from build123d import *

# Parameters (mm, degrees)
SKETCH1_R           = 3.5687
SKETCH1_R_2         = 2
BOSS_EXTRUDE1_DEPTH = 4.191
SKETCH5_R           = 2
SKETCH5_R_2         = 1.143
BOSS_EXTRUDE2_DEPTH = 0.2226
SKETCH6_R           = 0.5334
BOSS_EXTRUDE3_DEPTH = 1.524


with BuildPart() as part:
    # Sketch1 → Boss-Extrude1 (new body)
    with BuildSketch(Plane.XY.offset(-7.032965862)):
        with Locations((-5.5, 0)):
            Circle(SKETCH1_R)
        with Locations((-5.5, 0)):
            Circle(SKETCH1_R_2, mode=Mode.SUBTRACT)
    extrude(amount=BOSS_EXTRUDE1_DEPTH)

    # Sketch5 → Boss-Extrude2 (add)
    with BuildSketch(Plane.XY.offset(-4.232965862)):
        with Locations((-5.5, 0)):
            Circle(SKETCH5_R)
        with Locations((-5.5, 0)):
            Circle(SKETCH5_R_2, mode=Mode.SUBTRACT)
    extrude(amount=BOSS_EXTRUDE2_DEPTH)

    # Sketch6 → Boss-Extrude3 (add)
    with BuildSketch(Plane.XY.offset(-2.841965862)):
        with BuildLine():
            Line((-3.75375, -14.09065), (-2.68695, -2.195989387))
            ThreePointArc((-2.68695, -2.195989387), (-5.5, -3.5687), (-8.31305, -2.195989387))
            Line((-8.31305, -2.195989387), (-7.24625, -14.09065))
            ThreePointArc((-7.24625, -14.09065), (-5.5, -15.8369), (-3.75375, -14.09065))
        make_face()
        with Locations((-5.5, -12.92225)):
            Circle(SKETCH6_R, mode=Mode.SUBTRACT)
        with Locations((-5.5, -14.62405)):
            Circle(SKETCH6_R, mode=Mode.SUBTRACT)
        with Locations((-5.5, -11.22045)):
            Circle(SKETCH6_R, mode=Mode.SUBTRACT)
        with Locations((-5.5, -9.51865)):
            Circle(SKETCH6_R, mode=Mode.SUBTRACT)
        with Locations((-5.5, -7.81685)):
            Circle(SKETCH6_R, mode=Mode.SUBTRACT)
        with Locations((-5.5, -6.11505)):
            Circle(SKETCH6_R, mode=Mode.SUBTRACT)
    extrude(amount=-BOSS_EXTRUDE3_DEPTH)


solid = part.part
Input: part model. Units: mm. Frame: model coordinates. A direction names the side the tool comes from. Give positions to 0.01 mm unless a question says otherwise; leave off trailing zeros. Write each loop counter-clockwise with the first axis right and the second up, starting at its lowest first coordinate (ties: lowest second). Pieces come first, ordered by that corner, then holes. Notation, with made-up numbers: (30.5, 26) -> (51.5, 26) arc R8 cw to (51.5, 36) -> close; hole circle Ø1 at (-20, 11). An arc over 180 degrees is marked (long way). Use one line per item in the form item = value. Start each with the question number.
1) Pin query (flat end, axial travel): pin 1 (0.6 mm diameter, centred on x = -5.5, y = -11.22, fed in from +Z); pin 2 (1.7 mm diameter, centred on x = -5.5, y = -6.12, fed in from -Z); pin 3 (3 mm diameter, centred on x = -5.5, y = 0, fed in from +Z); pin 4 (1.5 mm diameter, centred on x = -6.5, z = -6, fed in from +Y). Return the tip coordinate at first contact, or that it passes through.
2) Draft query along X for faces 4 (the flat face through (-6, -9, -4.366)), 5 (the cylindrical face through (-5.96, 3.54, -4.97)), 6 (the cylindrical face through (-7.1, -1.2, -5.7)). Return one class per face: pulls with the +X half, pulls with the -X half, needs draft (parallel to the pull), parting line crosses it, or undercut.
3) Section query C-C on z = -5.25. Return the cut outline in (x, y), then the cut area to 3 significant figures.
4) Set-up query: faces 1 (the flat face through (-3.23, -8.23, -3.59)), 2 (the cylindrical face through (-7.1, -1.2, -3.4)), 3 (the flat face through (-5.5, -1.3, -4.233)). Return all of +Z, -Z, +X, -X, +Y, -Y with unobstructed straight access to the full face (end or side cutting, diameter ignored); none if empty.
5) Section query B-B on x = -6.25. Return the cut outline in (y, z), then the cut area to 3 significant figures.
6) Section query D-D on x = -5.5. Count the separate pieces of the cut face and the enclosed holes in it, then the cut area to 3 significant figures.
7) Section query A-A on y = 0. Return the cut outline in (x, z).
8) Ray query, probe 1 along Y at (x, z) = (-5.5, -6.2); probe 2 along X at (y, z) = (-14.5, -3.45); probe 3 along X at (y, z) = (1.75, -5.3). Return the intervals inside material, ascending. Write a range as from..to.
Outcome:
q1.pin_1 = through
q1.pin_2 = -4.37
q1.pin_3 = -4.01
q1.pin_4 = 3.56
q2.face_4 = needs draft
q2.face_5 = parting line crosses it
q2.face_6 = undercut
q3.outline = circle Ø7.14 at (-5.5, 0); hole circle Ø4 at (-5.5, 0)
q3.area = 27.4 mm^2
q4.face_1 = +Z, -Z, +X, -Y
q4.face_2 = +Z
q4.face_3 = -Z
q5.outline = (-15.67, -4.37) -> (-3.49, -4.37) -> (-3.49, -7.03) -> (-1.85, -7.03) -> (-1.85, -4.23) -> (-0.86, -4.23) -> (-0.86, -4.01) -> (-1.85, -4.01) -> (-1.85, -2.84) -> (-15.67, -2.84) -> close; (0.86, -4.23) -> (1.85, -4.23) -> (1.85, -7.03) -> (3.49, -7.03) -> (3.49, -2.84) -> (1.85, -2.84) -> (1.85, -4.01) -> (0.86, -4.01) -> close
q5.area = 32.7 mm^2
q6.separate_pieces = 8
q6.enclosed_holes = 0
q6.area = 22.5 mm^2
q7.outline = (-9.07, -7.03) -> (-7.5, -7.03) -> (-7.5, -4.23) -> (-6.64, -4.23) -> (-6.64, -4.01) -> (-7.5, -4.01) -> (-7.5, -2.84) -> (-9.07, -2.84) -> close; (-4.36, -4.23) -> (-3.5, -4.23) -> (-3.5, -7.03) -> (-1.93, -7.03) -> (-1.93, -2.84) -> (-3.5, -2.84) -> (-3.5, -4.01) -> (-4.36, -4.01) -> close
q8.probe_1 = -3.57..-2, 2..3.57
q8.probe_2 = -7.2..-6.02, -4.98..-3.8
q8.probe_3 = -8.61..-6.47, -4.53..-2.39
